from build123d import *

# Parameters (mm, degrees)
EXTRUDE_1_DEPTH     = 30
SKETCH_2_W          = 32
SKETCH_2_H          = 4
EXTRUDE_2_DEPTH     = 60
CUT_EXTRUDE_1_DEPTH = 30
SKETCH_6_W          = 4
SKETCH_6_H          = 32
EXTRUDE_4_DEPTH     = 20
SKETCH_7_W          = 4
SKETCH_7_H          = 60
EXTRUDE_5_DEPTH     = 32
SKETCH_8_R          = 3
CUT_EXTRUDE_3_DEPTH = 109
SKETCH_9_W          = 32
SKETCH_9_H          = 80
EXTRUDE_6_DEPTH     = 20
SKETCH_10_R         = 10
EXTRUDE_7_DEPTH     = 80
SKETCH_11_W         = 10
SKETCH_11_H         = 3
EXTRUDE_8_DEPTH     = 16
CUT_EXTRUDE_4_DEPTH = 16


with BuildPart() as part:
    # 草图1 → 凸台-拉伸1 (new body)
    with BuildSketch(Plane.XY):
        Polygon((-50, 16), (-16, 50), (16, 50), (50, 16), (50, -16), (46, -16), (46, 16), (16, 46), (-16, 46), (-46, 16), (-46, -16), (-50, -16), align=None)
    extrude(amount=EXTRUDE_1_DEPTH)

    # 草图2 → 凸台-拉伸2 (add)
    with BuildSketch(Plane(origin=(0, 0, 0), x_dir=(-1, 0, 0), z_dir=(0, 0, -1))):
        with Locations((0, 48)):
            Rectangle(SKETCH_2_W, SKETCH_2_H)
    extrude(amount=EXTRUDE_2_DEPTH)

    # 草图3 → 切除-拉伸1 (cut)
    with BuildSketch(Plane(origin=(0, 50, 0), x_dir=(1, 0, 0), z_dir=(0, 1, 0))):
        with BuildLine():
            Line((-16, 44), (-16, 67.226604698))
            Line((-16, 67.226604698), (16, 67.226604698))
            Line((16, 67.226604698), (16, 44))
            ThreePointArc((16, 44), (0, 60), (-16, 44))
        make_face()
    extrude(amount=-CUT_EXTRUDE_1_DEPTH, mode=Mode.SUBTRACT)

    # 草图6 → 凸台-拉伸4 (add)
    with BuildSketch(Plane.XY.offset(30)):
        with Locations((-48, 0)):
            Rectangle(SKETCH_6_W, SKETCH_6_H)
        with Locations((48, 0)):
            Rectangle(SKETCH_6_W, SKETCH_6_H)
    extrude(amount=EXTRUDE_4_DEPTH)

    # 草图7 → 凸台-拉伸5 (add)
    with BuildSketch(Plane(origin=(0, 16, 0), x_dir=(1, 0, 0), z_dir=(0, 1, 0))):
        with Locations((-52, -60)):
            Rectangle(SKETCH_7_W, SKETCH_7_H)
        with Locations((52, -60)):
            Rectangle(SKETCH_7_W, SKETCH_7_H)
    extrude(amount=-EXTRUDE_5_DEPTH)

    # 草图8 → 切除-拉伸3 (cut, through all)
    with BuildSketch(Plane.ZY.offset(54)):
        with Locations((74, 0)):
            Circle(SKETCH_8_R)
    extrude(amount=-CUT_EXTRUDE_3_DEPTH, mode=Mode.SUBTRACT)

    # 草图9 → 凸台-拉伸6 (add)
    with BuildSketch(Plane(origin=(0, 50, 0), x_dir=(1, 0, 0), z_dir=(0, 1, 0))):
        with Locations((0, -40)):
            Rectangle(SKETCH_9_W, SKETCH_9_H)
    extrude(amount=EXTRUDE_6_DEPTH)

    # 草图10 → 凸台-拉伸7 (add, symmetric)
    with BuildSketch(Plane(origin=(0, 0, 0), x_dir=(0, 0, -1), z_dir=(1, 0, 0))):
        with Locations((-70, 60)):
            Circle(SKETCH_10_R)
    extrude(amount=EXTRUDE_7_DEPTH, both=True)

    # 草图11 → 凸台-拉伸8 (add)
    with BuildSketch(Plane(origin=(50, 0, 0), x_dir=(0, 0, -1), z_dir=(1, 0, 0))):
        with Locations((-15, -3.5)):
            Rectangle(SKETCH_11_W, SKETCH_11_H)
        with Locations((-15, 3.5)):
            Rectangle(SKETCH_11_W, SKETCH_11_H)
    extrude(amount=EXTRUDE_8_DEPTH)

    # 草图12 → 切除-拉伸4 (cut)
    with BuildSketch(Plane(origin=(0, 5, 0), x_dir=(1, 0, 0), z_dir=(0, 1, 0))):
        with BuildLine():
            Line((61, -10), (68.714035349, -10))
            Line((68.714035349, -10), (68.714035349, -20))
            Line((68.714035349, -20), (61, -20))
            ThreePointArc((61, -20), (66, -15), (61, -10))
        make_face()
    extrude(amount=-CUT_EXTRUDE_4_DEPTH, mode=Mode.SUBTRACT)


solid = part.part
Input: part model. Units: mm. Frame: model coordinates. A direction names the side the tool comes from. Coordinates: 2 decimals unless noted, no trailing zeros. Loops run counter-clockwise (first coordinate to the right, second up) from the corner with the lowest first, then second, coordinate; pieces in that order, holes last.
Q1. Contact query for flat-ended pins moving along their axis: pin 1 (1.2 mm diameter, centred on x = 47.5, y = 1, fed in from +Z); pin 2 (4 mm diameter, centred on y = -4, z = 21, fed in from +X); pin 3 (1 mm diameter, centred on y = 6, z = 46, fed in from +X); pin 4 (5 mm diameter, centred on y = 0, z = 74, fed in from +X). Output: stop coordinate, or through.
Q2. Cut plane B-B (y = 36). Output: boundary loops of the cut face in (x, z), then the cut area to 3 significant figures.
Q3. Material intervals for line 1 (X direction, y = 5, z = 70.5); line 2 (Y direction, x = 52, z = 74); line 3 (Y direction, x = 15, z = -7), sorted ascending.
Q4. Cut plane A-A (y = 0). Output: boundary loops of the cut face in (x, z).
Q5. Cut plane D-D (x = 22). Output: boundary loops of the cut face in (y, z), then the cut area to 3 significant figures.
Q6. Cut plane C-C (z = 67.5). Output: boundary loops of the cut face in (x, y).
Q7. Draft query along X for faces 1 (the face through (-52, 0, 30)), 2 (the face through (-33, 33, 15)), 3 (the face through (-46, 0, 25)), 4 (the face through (-50, 0, 70)). Return one class per face: +X half, -X half, draft (parallel to the pull), parting line (faces both ways), or undercut.
Q8. Set-up query: faces 5 (the face through (51, 16, 53)), 6 (the face through (-16, 48, -22)), 7 (the face through (48, 0, 50)). Return all of +Z, -Z, +X, -X, +Y, -Y with unobstructed straight access to the full face (end or side cutting, diameter ignored); none if empty.
Working result:
1. pin 1: stops at z = 50
1. pin 2: stops at x = 64
1. pin 3: stops at x = 54
1. pin 4: passes through
2. outline: (-30, 0) - (-26, 0) - (-26, 30) - (-30, 30) - close; (26, 0) - (30, 0) - (30, 30) - (26, 30) - close
2. area: 240 mm2
3. line 1: x = -54 to -50, 50 to 54
3. line 2: y = -16 to -3, 3 to 16, 50.83 to 69.17
3. line 3: y = 46 to 50
4. outline: (-54, 30) - (-50, 30) - (-50, 0) - (-46, 0) - (-46, 50) - (-50, 50) - (-50, 71) - (-54, 71) - close; (-54, 77) - (-50, 77) - (-50, 90) - (-54, 90) - close; (46, 0) - (50, 0) - (50, 30) - (54, 30) - (54, 71) - (50, 71) - (50, 50) - (46, 50) - close; (50, 77) - (54, 77) - (54, 90) - (50, 90) - close
5. outline: (40, 0) - (44, 0) - (44, 30) - (40, 30) - close; circle Ø20 at (60, 70)
5. area: 434 mm2
6. outline: (-80, 50.32) - (-16, 50.32) - (-16, 50) - (16, 50) - (16, 50.32) - (80, 50.32) - (80, 69.68) - (16, 69.68) - (16, 70) - (-16, 70) - (-16, 69.68) - (-80, 69.68) - close; (-54, -16) - (-50, -16) - (-50, 16) - (-54, 16) - close; (50, -16) - (54, -16) - (54, 16) - (50, 16) - close
7. face 1: draft
7. face 2: -X half
7. face 3: undercut
7. face 4: undercut
8. face 5: +Z, +X, -X
8. face 6: -Z, -X, +Y, -Y
8. face 7: +Z, +Y, -Y
